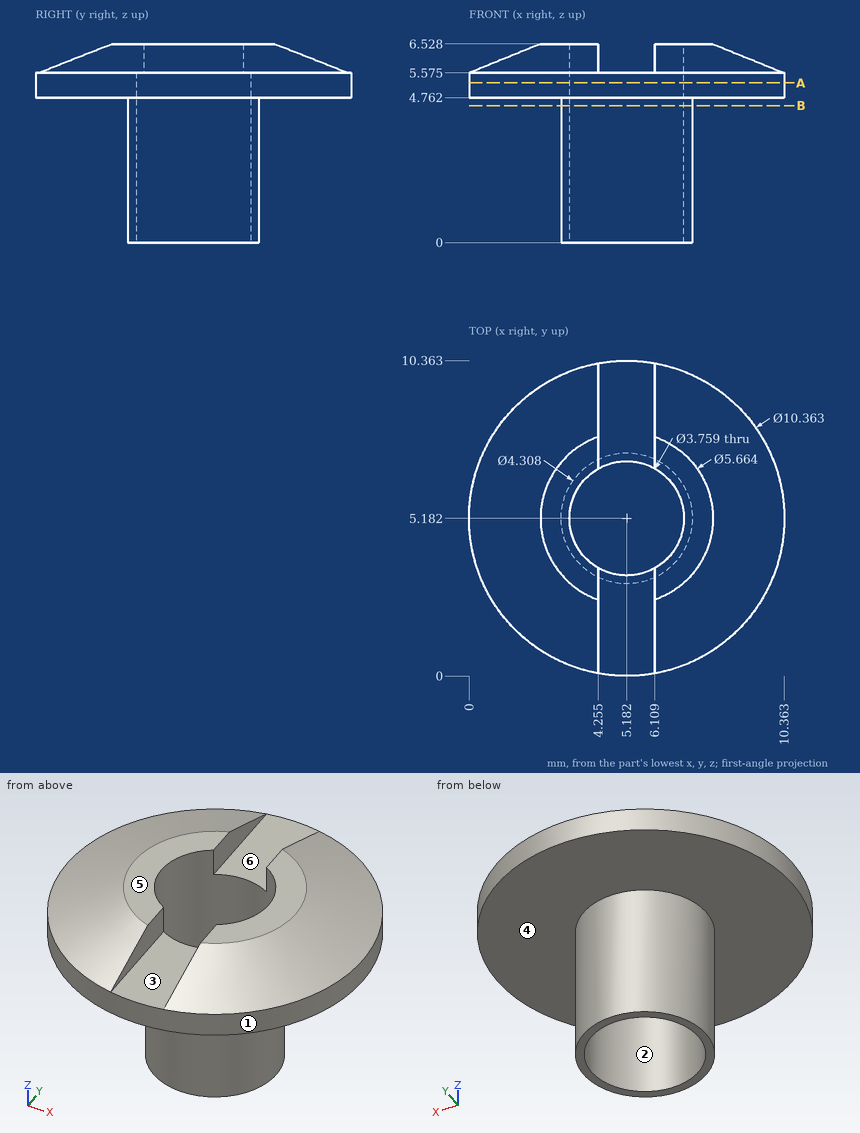
Study the drawing (mm; zero at the part's minimum x, y, z) and answer. A direction names the side the tool comes from. Coordinates: 2 decimals unless noted, no trailing zeros. Order: outer loops, then holes, each group sorted by start corner. A loop starts at its lowest first (then second) coordinate and runs counter-clockwise, first axis right, second up. Notation, with made-up numbers: M 14,-1.5 L 40,-1.5 A20 ccw 40,5.5 Z; hole C 42,-11 d4. An arc over 180 degrees is marked long. Answer as a JSON object with one key per item and string values. Group by question number.
1. Section A-A on z = 5.25 is taken. Write down the section's boundary in (x, y).
2. A flat-ended cylindrical pin translates along its axis: P1, Ø0.9, axis at x = 5, y = 1.5, coming from the +Z side (1 decimal). Find the tip coordinate at first contact, or state that the pin passes through.
3. Determine the mould class of the marked faces 1, 2 and 3 for opening direction Y: released by +Y, released by -Y, zero draft, split by the parting line, or undercut.
4. Straight lines are drawn through the part: line 1 (Y direction, x = 5.25, z = 2.75) (1 decimal); line 2 (Z direction, x = 5.75, y = 9.25) (1 decimal). For each, find the intervals that lie inside material, in ascending order.
5. Section B-B on z = 4.5 is taken. Write down the section's boundary in (x, y) (1 decimal).
6. A tool of negligible diameter and unlimited length cuts with its end or side. For the marked faces 4, 5 and 6, from which of +Z, -Z, +X, -X, +Y, -Y can it reach the whole face along a straight path? Write none if from no direction.
Values follow:
{
 "1": {"outline": "C 5.18,5.18 d10.36; hole C 5.18,5.18 d3.76"},
 "2": {"P1": "z = 5.6"},
 "3": {"face 1": "split by the parting line", "face 2": "undercut", "face 3": "zero draft"},
 "4": {"line 1": "3 to 3.3, 7.1 to 7.3", "line 2": "4.8 to 5.6"},
 "5": {"outline": "C 5.2,5.2 d4.3; hole C 5.2,5.2 d3.8"},
 "6": {"face 4": "-Z", "face 5": "+Z, +X, -X, +Y, -Y", "face 6": "+Z, +Y, -Y"}
}
